Verification items for the finished model (mm, model axes). Face numbers are marked on the shaded views. A direction names the side the tool comes from. Coordinates: 2 decimals unless noted, no trailing zeros. Loops run counter-clockwise (first coordinate to the right, second up) from the corner with the lowest first, then second, coordinate; pieces in that order, holes last. Notation, with made-up numbers: (18, 77.5) - (49, 77.5) arc R18 ccw to (49, 87.5) - close; hole circle Ø3 at (-3, 51). An arc over 180 degrees is marked (long way). One line per item, written item: value. Start each with the question number.
(1) Draft check along X on the marked faces 4, 5 and 6. Enter one of: +X half, -X half, draft (parallel to the pull), parting line (faces both ways), or undercut.
(2) Thickness scan on probe 1 along Y at (x, z) = (0, -0.5); probe 2 along Y at (x, z) = (0, 24); probe 3 along Z at (x, y) = (-28, -27). Record the ranges inside material, lowest first. Write a range as [from, to].
(3) Set-up check for the marked faces 1, 2 and 3: record each of +Z, -Z, +X, -X, +Y, -Y from which the full face is reachable in a straight line by a thin tool's end or side.
(4) Gauge pin test, flat ends, axial feed: P1, Ø1.5, axis at y = 30.5, z = 20, coming from the +X side; P2, Ø3, axis at y = 47.5, z = 10.5, coming from the -X side; P3, Ø5, axis at x = -46.5, z = 14, coming from the +Y side. Record the tip position at first contact, or that the pin passes through.
(5) Section check B-B (x = 0). Count the separate pieces of the cut face and the enclosed holes in it, plus the area to 3 significant figures.
(6) Section check C-C (x = 39.5). Record the boundary of the cut face in (y, z).
(7) Section check A-A (z = 19.25). Record the boundary of the cut face in (x, y), plus the area to 3 significant figures.
```python
from build123d import *

# Parameters (mm, degrees)
F0_R     = 51.0634311227
F0_R_2   = 44.6472785168
F1_DEPTH = 25
F2_R     = 51.658363485
F3_DEPTH = 3
F4_W     = 8.4723439068
F4_H     = 17.9225206375
F5_DEPTH = 87.2
F6_W     = 8.4723439068
F6_H     = 17.9225206375
F7_DEPTH = 61.9
F8_R     = 1.5
F9_DEPTH = 28.001


with BuildPart() as f1:
    # F0 (on Top) → F1 (new body)
    with BuildSketch(Plane.XY):
        Circle(F0_R)
        Circle(F0_R_2, mode=Mode.SUBTRACT)
    extrude(amount=F1_DEPTH)

    # F2 (on face) → F3 (join)
    with BuildSketch(Plane(origin=(0, 0, 0), x_dir=(1, 0, 0), z_dir=(0, 0, -1))):
        Circle(F2_R)
    extrude(amount=F3_DEPTH)

    # F4 (on Front) → F5 (cut, symmetric)
    with BuildSketch(Plane.XZ):
        with Locations((0, 12.7205625176)):
            Rectangle(F4_W, F4_H)
    extrude(amount=F5_DEPTH, both=True, mode=Mode.SUBTRACT)

    # F6 (on Right) → F7 (cut, symmetric)
    with BuildSketch(Plane.YZ):
        with Locations((0, 12.8065040335)):
            Rectangle(F6_W, F6_H)
    extrude(amount=F7_DEPTH, both=True, mode=Mode.SUBTRACT)

    # F8 (on face) → F9 (cut, through all)
    with BuildSketch(Plane.XY.offset(25)):
        with Locations((0, 48.2453033328)):
            Circle(F8_R)
        with Locations((0, -48.2453033328)):
            Circle(F8_R)
        with Locations((-48.2453033328, 0)):
            Circle(F8_R)
        with Locations((48.2453033328, 0)):
            Circle(F8_R)
    extrude(amount=-F9_DEPTH, mode=Mode.SUBTRACT)


solid = f1.part
```
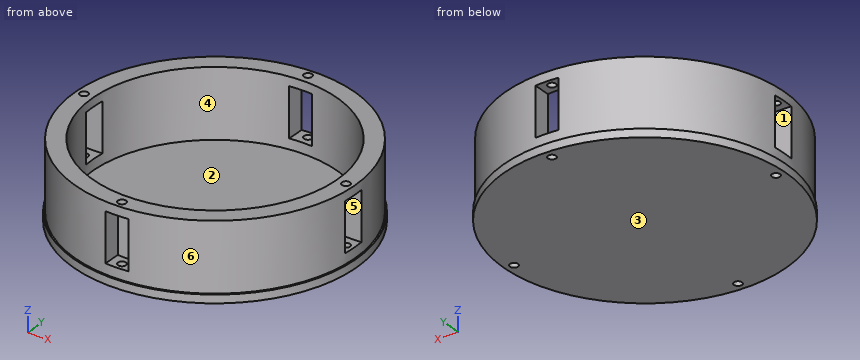
Responses:
1. face 4: undercut
1. face 5: draft
1. face 6: parting line
2. probe 1: y = [-51.66, -49.75], [-46.75, 46.75], [49.75, 51.66]
2. probe 2: y = [-51.06, -49.75], [-46.75, -44.65], [44.65, 46.75], [49.75, 51.06]
2. probe 3: z = [-3, 0]
3. face 1: +X, -X
3. face 2: +Z
3. face 3: -Z, +X, -X, +Y, -Y
4. P1: stops at x = 41.5
4. P2: stops at x = -22.17
4. P3: stops at y = 25.91
5. separate pieces: 7
5. enclosed holes: 0
5. area: 340 mm²
6. outline: (-33.29, -3) - (33.29, -3) - (33.29, 0) - (32.36, 0) - (32.36, 25) - (20.81, 25) - (20.81, 0) - (-20.81, 0) - (-20.81, 25) - (-32.36, 25) - (-32.36, 0) - (-33.29, 0) - close
7. outline: (-50.89, -4.24) arc R51.06 ccw to (-4.24, -50.89) - (-4.24, -44.45) arc R44.65 cw to (-44.45, -4.24) - close; (-50.89, 4.24) - (-44.45, 4.24) arc R44.65 cw to (-4.24, 44.45) - (-4.24, 50.89) arc R51.06 ccw to start; (4.24, -50.89) arc R51.06 ccw to (50.89, -4.24) - (44.45, -4.24) arc R44.65 cw to (4.24, -44.45) - close; (4.24, 44.45) arc R44.65 cw to (44.45, 4.24) - (50.89, 4.24) arc R51.06 ccw to (4.24, 50.89) - close
7. area: 1,710 mm²
